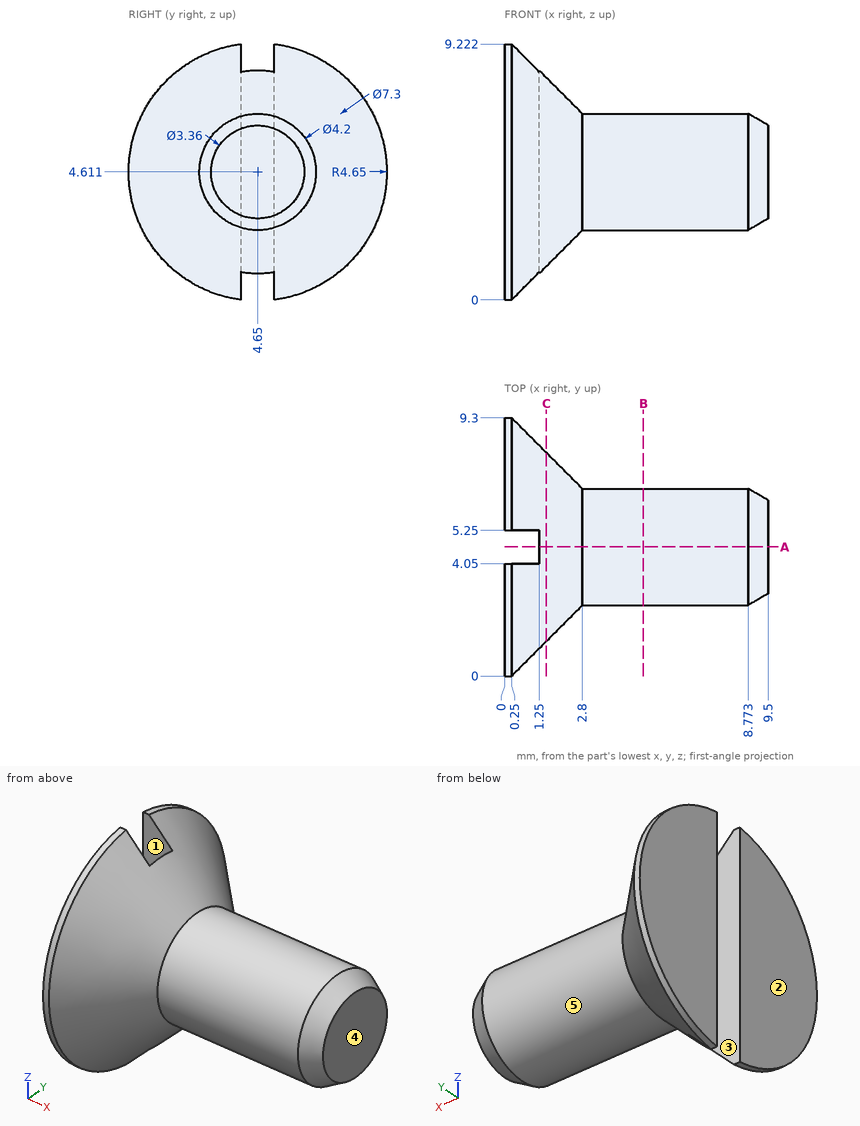
For this review, use the dimensioned drawing (mm, ordinates from the lowest corner) and the shaded views. A direction names the side the tool comes from. Coordinates: 2 decimals unless noted, no trailing zeros. Order: outer loops, then holes, each group sorted by start corner. A loop starts at its lowest first (then second) coordinate and runs counter-clockwise, first axis right, second up. Notation, with made-up numbers: (27, 71) - (35, 71) arc R15 cw to (35, 83) - close; hole circle Ø11 at (0.25, 24.25). An arc over 180 degrees is marked (long way). Answer in a Markdown table with one row per item.
(1) Consider section C-C on x = 1.5. State the section outline as (y, z) points.
Checked values:
| item | result |
|---|---|
| outline | circle Ø6.8 at (4.65, 4.61) |
(2) Consider section B-B on x = 5. State the section outline as (y, z) points.
Checked values:
| item | result |
|---|---|
| outline | circle Ø4.2 at (4.65, 4.61) |
(3) Wall thickness on line 1 along Y through (x, z) = (1, 8); line 2 along X through (y, z) = (1, 7.25) (1 decimal); line 3 along Y through (x, z) = (8, 6) (1 decimal): over which ranges is each line inside the solid? List them lowest first. Write a range as from..to.
Checked values:
| item | result |
|---|---|
| line 1 | 2.72..4.05, 5.25..6.58 |
| line 2 | 0..0.4 |
| line 3 | 3.1..6.2 |
(4) For the marked faces 1 and 2, list the 3-axis set-ups (+Z, -Z, +X, -X, +Y, -Y) from which the entire face can be reached by the end or side of a thin tool; tool diameter is ignored.
Checked values:
| item | result |
|---|---|
| face 1 | +Z, -Z, -X |
| face 2 | +Z, -Z, -X, +Y, -Y |
(5) The part is to be moulded in two halves that separate along Y. For the marked faces 3, 4 and 5, say which applies: released by +Y, released by -Y, zero draft, split by the parting line, or undercut.
Checked values:
| item | result |
|---|---|
| face 3 | undercut |
| face 4 | zero draft |
| face 5 | split by the parting line |
(6) Consider section A-A on y = 4.65. State the section outline as (x, z) points.
Checked values:
| item | result |
|---|---|
| outline | (1.25, 0.96) - (2.8, 2.51) - (8.77, 2.51) - (9.5, 2.93) - (9.5, 6.29) - (8.77, 6.71) - (2.8, 6.71) - (1.25, 8.26) - close |
(7) Clearance check with flat-ended pins moving along their axes: pin 1 (4 mm diameter, centred on y = 6.5, z = 3.5, fed in from +X); pin 2 (1.5 mm diameter, centred on x = 7, y = 4.5, fed in from +Z); pin 3 (1 mm diameter, centred on x = 0.5, z = 4, fed in from -Y). State where each tip first meets the part, or that it passes through.
Checked values:
| item | result |
|---|---|
| pin 1 | x = 9.5 |
| pin 2 | z = 6.71 |
| pin 3 | y = 0 |
